Geometry check sheet. Reference: the model listing, model coordinates, mm. Coordinates: 2 decimals unless noted, no trailing zeros. Loops run counter-clockwise (first coordinate to the right, second up) from the corner with the lowest first, then second, coordinate; pieces in that order, holes last. Notation, with made-up numbers: (-3, 89) - (26, 89) arc R18 cw to (26, 122) - close; hole circle Ø4 at (82, 46.5). An arc over 180 degrees is marked (long way). One line per item, written item: value.
from build123d import *

# Parameters (mm, degrees)
PAD_DEPTH    = 10
THICKNESS_T  = -1
SKETCH001_R  = 2.5
POCKET_DEPTH = 10.001


with BuildPart() as part:
    # Sketch → Pad (new body)
    with BuildSketch(Plane.XZ):
        Polygon((-5, 0), (5, 0), (5, 104.4084), (16.620565, 152.82742), (31, 172), (23, 178), (7.379435, 157.17258), (-5, 105.5916), align=None)
    extrude(amount=PAD_DEPTH)

    # Thickness
    thickness_openings = [part.faces().sort_by_distance(p)[0] for p in [
        (27, -5, 175),
        (0, -5, 0),
    ]]
    offset(amount=THICKNESS_T, openings=thickness_openings)

    # Sketch001 (on Face8 of Thickness) → Pocket (cut, through all)
    with BuildSketch(Plane.XZ.offset(10)):
        with Locations((0, 5)):
            Circle(SKETCH001_R)
        with Locations((12, 155)):
            Circle(SKETCH001_R)
        with Locations((24, 171)):
            Circle(SKETCH001_R)
    extrude(amount=-POCKET_DEPTH, mode=Mode.SUBTRACT)


solid = part.part
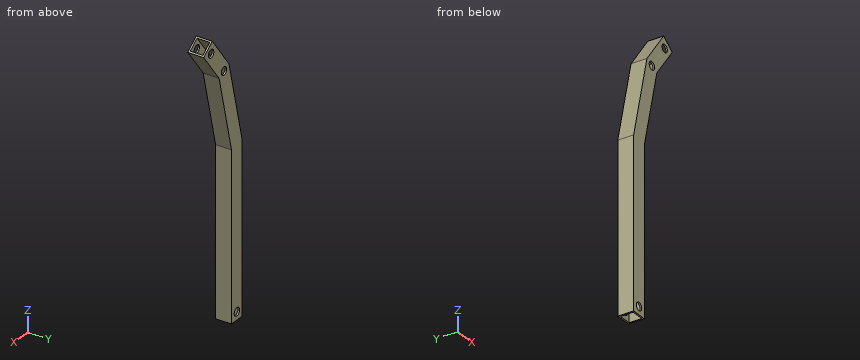
(1) Cross-section at A-A on y = -7. Record the cut outline in (x, z), and give its area (3 significant figures).
Reply:
outline: (-5, 0) - (-4, 0) - (-4, 105.47) - (8.3, 156.74) - (23.8, 177.4) - (23, 178) - (7.38, 157.17) - (-5, 105.59) - close; (4, 0) - (5, 0) - (5, 104.41) - (16.62, 152.83) - (31, 172) - (30.2, 172.6) - (15.82, 153.43) arc R1 ccw to (15.65, 153.06) - (4.03, 104.64) arc R1 ccw to (4, 104.41) - close
area: 363 mm2
(2) Cross-section at C-C on x = 12. Record the cut outline in (y, z), and give its area (3 significant figures).
Reply:
outline: (-10, 133.58) - (0, 133.58) - (0, 152.5) - (-1, 152.5) - (-1, 137.86) - (-9, 137.86) - (-9, 152.5) - (-10, 152.5) - close; (-10, 157.5) - (-9, 157.5) - (-9, 161.67) - (-1, 161.67) - (-1, 157.5) - (0, 157.5) - (0, 163.33) - (-10, 163.33) - close
area: 97.1 mm2
(3) Go/stop test with flat-tipped pins: pin 1 Ø4.5 at (x, z) = (0, 5) entering from -Y; pin 2 Ø5 at (y, z) = (-3.5, 47) entering from +X; pin 3 Ø5 at (x, y) = (20, -3.5) entering from -Z; pin 4 Ø2 at (x, y) = (26, -7) entering from -Z. Record where each tip stops, or that it passes through.
Reply:
pin 1: through
pin 2: x = 5
pin 3: z = 154
pin 4: z = 164
(4) Cross-section at D-D on z = 5. Record the cut outline in (x, y).
Reply:
outline: (-5, -10) - (-2.5, -10) - (-2.5, -9) - (-4, -9) - (-4, -1) - (-2.5, -1) - (-2.5, 0) - (-5, 0) - close; (2.5, -10) - (5, -10) - (5, 0) - (2.5, 0) - (2.5, -1) - (4, -1) - (4, -9) - (2.5, -9) - close
(5) Material ranges on probe 1 along X at (y, z) = (-1.75, 96); probe 2 along Y at (x, z) = (2, 41.5); probe 3 along X at (y, z) = (-0.75, 43), recorded low to high. Write a range as from..to.
Reply:
probe 1: -5..-4, 4..5
probe 2: -10..-9, -1..0
probe 3: -5..5
(6) Cross-section at B-B on z = 32. Record the cut outline in (x, y).
Reply:
outline: (-5, -10) - (5, -10) - (5, 0) - (-5, 0) - close; hole (-4, -9) - (4, -9) - (4, -1) - (-4, -1) - close
